For this review, use the dimensioned drawing (mm, ordinates from the lowest corner) and the shaded views. A direction names the side the tool comes from. Round coordinates to 2 decimals unless told otherwise and drop trailing zeros. Write each loop counter-clockwise with the first axis right and the second up, starting at its lowest first coordinate (ties: lowest second). Pieces come first, ordered by that corner, then holes. Notation, with made-up numbers: (61, 3) - (120, 3) arc R27 cw to (120, 21) - close; hole circle Ø6 at (72, -8.5). An arc over 180 degrees is marked (long way). Return JSON: item names as keys, results as strings.
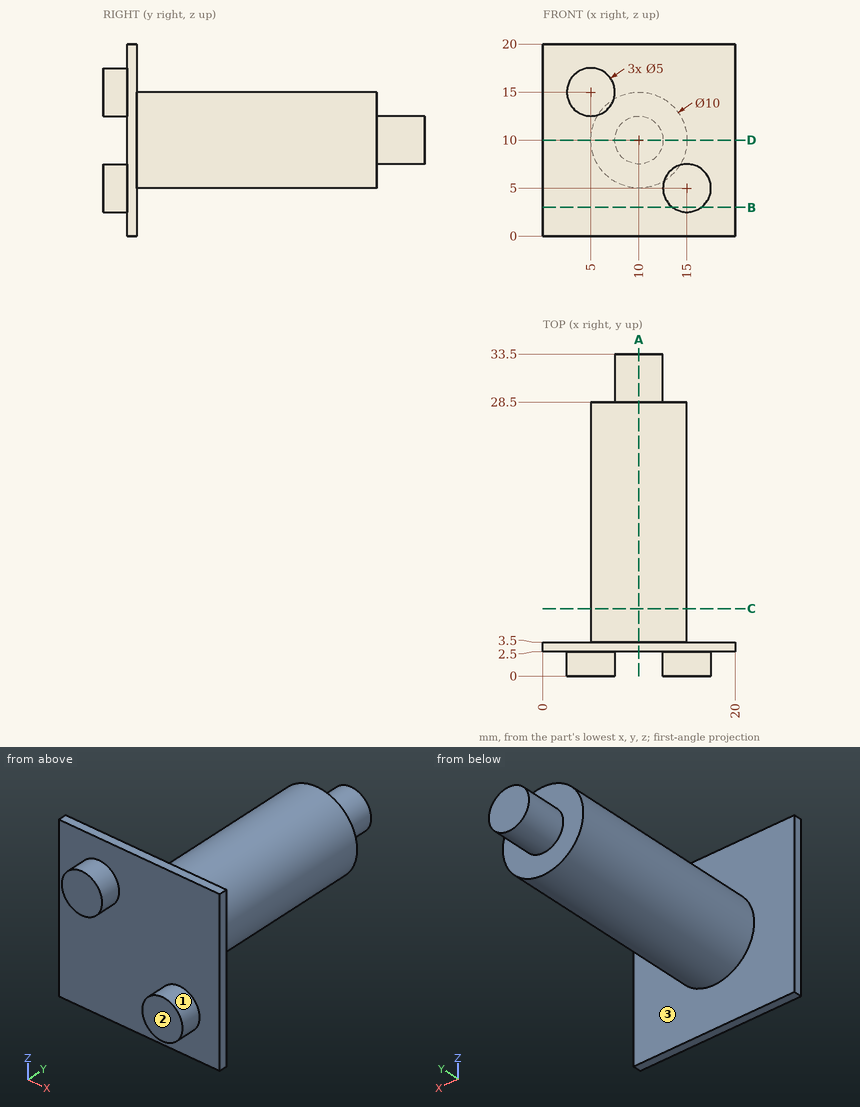
(1) For the marked faces 1, 2 and 3, list the 3-axis set-ups (+Z, -Z, +X, -X, +Y, -Y) from which the entire face can be reached by the end or side of a thin tool; tool diameter is ignored.
Filled in:
{"face 1": "-Y", "face 2": "+Z, -Z, +X, -X, -Y", "face 3": "+Y"}
(2) Add section D-D (z = 10). Write out the cut boundary in (x, y).
Filled in:
{"outline": "(0, 2.5) - (20, 2.5) - (20, 3.5) - (15, 3.5) - (15, 28.5) - (12.5, 28.5) - (12.5, 33.5) - (7.5, 33.5) - (7.5, 28.5) - (5, 28.5) - (5, 3.5) - (0, 3.5) - close"}
(3) Add section C-C (y = 7). Write out the cut boundary in (x, z).
Filled in:
{"outline": "circle Ø10 at (10, 10)"}
(4) Add section A-A (x = 10). Write out the cut boundary in (y, z), plus the area to 3 significant figures.
Filled in:
{"outline": "(2.5, 0) - (3.5, 0) - (3.5, 5) - (28.5, 5) - (28.5, 7.5) - (33.5, 7.5) - (33.5, 12.5) - (28.5, 12.5) - (28.5, 15) - (3.5, 15) - (3.5, 20) - (2.5, 20) - close", "area": "295 mm2"}
(5) Clearance check with flat-ended pins moving along their axes: pin 1 Ø5 at (x, y) = (17, 14) entering from +Z; pin 2 Ø2 at (y, z) = (9, 9.5) entering from -X; pin 3 Ø10 at (x, y) = (12.5, 30) entering from +Z. State where each tip first meets the part, or that it passes through.
Filled in:
{"pin 1": "stops at z = 12.18", "pin 2": "stops at x = 5", "pin 3": "stops at z = 15"}
(6) Wall thickness on line 1 (Y direction, x = 9.75, z = 16.5); line 2 (Y direction, x = 5.75, z = 16.5); line 3 (X direction, y = 26, z = 10.25): over which ranges is each line inside the solid? List them lowest first.
Filled in:
{"line 1": "y = 2.5 to 3.5", "line 2": "y = 0 to 3.5", "line 3": "x = 5.01 to 14.99"}
(7) Add section B-B (z = 3). Write out the cut boundary in (x, y), plus the area to 3 significant figures.
Filled in:
{"outline": "(0, 2.5) - (13.5, 2.5) - (13.5, 0) - (16.5, 0) - (16.5, 2.5) - (20, 2.5) - (20, 3.5) - (0, 3.5) - close", "area": "27.5 mm2"}
